The listing builds one solid part. Answer for the finished solid, in the listing's coordinates (mm). A direction names the side the tool comes from. Give positions to 0.01 mm unless a question says otherwise; leave off trailing zeros. Order: outer loops, then holes, each group sorted by start corner. A loop starts at its lowest first (then second) coordinate and runs counter-clockwise, first axis right, second up. Notation, with made-up numbers: (-39.5, 67.25) - (4.5, 67.25) arc R21 cw to (4.5, 92.25) - close; hole circle Ø1 at (-25, 37.25). An arc over 180 degrees is marked (long way). Use CSV: the item, a comma, the result in double quotes.
```python
from build123d import *

# Parameters (mm, degrees)
CUT_EXTRUDE1_START = -2.54
SKETCH2_R          = 10.195320638
SKETCH2_R_2        = 6.35
CUT_EXTRUDE1_DEPTH = 2.54


with BuildPart() as part:
    # Sketch1 → Revolve1 (revolve)
    with BuildSketch(Plane(origin=(0, 0, 0), x_dir=(0, 0, -1), z_dir=(1, 0, 0)), mode=Mode.PRIVATE) as revolve1_sk:
        Polygon((0, 0), (0, 10.16), (12.7, 10.16), (12.7, 6.35), (26.9875, 6.35), (26.9875, 0), align=None)
    revolve(revolve1_sk.sketch.rotate(Axis((0, 0, 0), (0, 0, -1)), 90), axis=Axis((0, 0, 0), (0, 0, -1)))

    # Sketch2 → Cut-Extrude1 (cut)
    with BuildSketch(Plane.XY.offset(CUT_EXTRUDE1_START)):
        Circle(SKETCH2_R)
        Circle(SKETCH2_R_2, mode=Mode.SUBTRACT)
    extrude(amount=CUT_EXTRUDE1_DEPTH, mode=Mode.SUBTRACT)


solid = part.part
```
Item 1: Which of the six approach directions +Z, -Z, +X, -X, +Y, -Y give full straight-line access (tool end or side, diameter ignored) to faces 1 (the face through (-1.38, -6.2, -1.29)), 2 (the face through (-1.323, -10.074, -7.691)), 3 (the face through (0, 7, -12.7))?
Taken from the geometry:
face 1,"+Z"
face 2,"+Z, -Z"
face 3,"-Z"
Item 2: The part is cut by section D-D (z = -20.5). Give the vertices of the cut face in (x, y), and give its area (3 significant figures).
Taken from the geometry:
outline,"circle Ø12.7 at (0, 0)"
area,"127 mm^2"
Item 3: The part is cut by section A-A (y = 0). Give the vertices of the cut face in (x, z), and give its area (3 significant figures).
Taken from the geometry:
outline,"(-10.16, -12.7) - (-6.35, -12.7) - (-6.35, -26.99) - (6.35, -26.99) - (6.35, -12.7) - (10.16, -12.7) - (10.16, -2.54) - (6.35, -2.54) - (6.35, 0) - (-6.35, 0) - (-6.35, -2.54) - (-10.16, -2.54) - close"
area,"420 mm^2"
Item 4: The part is cut by section C-C (z = -7). Give the vertices of the cut face in (x, y).
Taken from the geometry:
outline,"circle Ø20.32 at (0, 0)"
Item 5: Find the intervals of material crossed by line 1 along Z through (x, y) = (6.25, 6.5); line 2 along Y through (x, z) = (0.25, -25); line 3 along X through (y, z) = (9, -9), in increasing order.
Taken from the geometry:
line 1,"-12.7 to -2.54"
line 2,"-6.35 to 6.35"
line 3,"-4.71 to 4.71"
Item 6: Each of these flat-tipped pins is pushed along its axis until it touches: pin 1 (6 mm diameter, centred on x = -4, z = -4.5, fed in from -Y); pin 2 (6 mm diameter, centred on y = 4.5, z = -22.5, fed in from +X); pin 3 (5 mm diameter, centred on x = 8, z = -20, fed in from +Y). Where does it stop, or does it pass through?
Taken from the geometry:
pin 1,"y = -10.11"
pin 2,"x = 6.17"
pin 3,"y = 3.17"
